from build123d import *

# Parameters (mm, degrees)
SKETCH2_W               = 7.62
SKETCH2_H               = 7.62
BOSS_EXTRUDE1_DEPTH     = 12.7
F_8_CLEARANCE_HOLE1_D   = 4.9149
CUT_EXTRUDE1_REACH      = 27.965
CUT_EXTRUDE1_END_RADIUS = 3.47345
SKETCH5_W               = 3.175
SKETCH5_H               = 3.175
CUT_EXTRUDE2_REACH      = 27.965
CUT_EXTRUDE2_END_RADIUS = 3.47345
CUT_EXTRUDE3_REACH      = 27.965
CUT_EXTRUDE3_END_RADIUS = 3.47345
SKETCH7_W               = 3.575
SKETCH7_H               = 3.575
SKETCH7_W_2             = 3.175
SKETCH7_H_2             = 3.175
CUT_EXTRUDE4_REACH      = 27.965
CUT_EXTRUDE4_END_RADIUS = 3.47345


with BuildPart() as part:
    # Sketch2 → Boss-Extrude1 (new, symmetric)
    with BuildSketch(Plane.XY):
        Rectangle(SKETCH2_W, SKETCH2_H)
    extrude(amount=BOSS_EXTRUDE1_DEPTH, both=True)

    # #8 Clearance Hole1 (through all)
    with Locations(Plane(origin=(0, 3.81, 0), x_dir=(1, 0, 0), z_dir=(0, 1, 0))):
        with Locations((0, 0)):
            Hole(F_8_CLEARANCE_HOLE1_D / 2)

    # Cut-Extrude1: up to this cylinder (the profile starts outside it)
    cut_extrude1_end = Plane(origin=(0, 0, 0), z_dir=(0, 1, 0)) * Cylinder(CUT_EXTRUDE1_END_RADIUS, 63.8769, mode=Mode.PRIVATE)
    # Sketch5 → Cut-Extrude1 (cut, up to the surface)
    with BuildSketch(Plane.XY.offset(12.7), mode=Mode.PRIVATE) as cut_extrude1_sk1:
        Rectangle(SKETCH5_W, SKETCH5_H)
    cut_extrude1_tool1 = extrude(cut_extrude1_sk1.sketch, amount=-CUT_EXTRUDE1_REACH, mode=Mode.PRIVATE) - cut_extrude1_end
    add(cut_extrude1_tool1.solids().sort_by_distance((0, 0, 12.7))[0], mode=Mode.SUBTRACT)

    # Cut-Extrude2: up to this cylinder (the profile starts outside it)
    cut_extrude2_end = Plane(origin=(0, 0, 0), z_dir=(0, 1, 0)) * Cylinder(CUT_EXTRUDE2_END_RADIUS, 63.8769, mode=Mode.PRIVATE)
    # Sketch6 → Cut-Extrude2 (cut, up to the surface)
    with BuildSketch(Plane(origin=(0, 0, -12.7), x_dir=(-1, 0, 0), z_dir=(0, 0, -1)), mode=Mode.PRIVATE) as cut_extrude2_sk1:
        with BuildLine():
            Line((1.499999936, 1.322875825), (1.499999936, -1.322875825))
            ThreePointArc((1.499999936, -1.322875825), (-2.000000064, 0), (1.499999936, 1.322875825))
        make_face()
    cut_extrude2_tool1 = extrude(cut_extrude2_sk1.sketch, amount=-CUT_EXTRUDE2_REACH, mode=Mode.PRIVATE) - cut_extrude2_end
    add(cut_extrude2_tool1.solids().sort_by_distance((0.132366, 0, -12.7))[0], mode=Mode.SUBTRACT)

    # Cut-Extrude3: up to this cylinder (the profile starts outside it)
    cut_extrude3_end = Plane(origin=(0, 0, 0), z_dir=(0, 1, 0)) * Cylinder(CUT_EXTRUDE3_END_RADIUS, 63.8769, mode=Mode.PRIVATE)
    # Sketch7 → Cut-Extrude3 (cut, up to the surface)
    with BuildSketch(Plane.XY.offset(12.7), mode=Mode.PRIVATE) as cut_extrude3_sk1:
        Rectangle(SKETCH7_W, SKETCH7_H)
        Rectangle(SKETCH7_W_2, SKETCH7_H_2, mode=Mode.SUBTRACT)
    cut_extrude3_tool1 = extrude(cut_extrude3_sk1.sketch, amount=-CUT_EXTRUDE3_REACH, mode=Mode.PRIVATE) - cut_extrude3_end
    add(cut_extrude3_tool1.solids().sort_by_distance((-1.736942, 0, 12.7))[0], mode=Mode.SUBTRACT)

    # Cut-Extrude4: up to this cylinder (the profile starts outside it)
    cut_extrude4_end = Plane(origin=(0, 0, 0), z_dir=(0, 1, 0)) * Cylinder(CUT_EXTRUDE4_END_RADIUS, 63.8769, mode=Mode.PRIVATE)
    # Sketch8 → Cut-Extrude4 (cut, up to the surface)
    with BuildSketch(Plane(origin=(0, 0, -12.7), x_dir=(-1, 0, 0), z_dir=(0, 0, -1)), mode=Mode.PRIVATE) as cut_extrude4_sk1:
        with BuildLine():
            Line((1.699999936, -1.396424183), (1.699999936, 1.396424183))
            ThreePointArc((1.699999936, 1.396424183), (-2.200000064, 0), (1.699999936, -1.396424183))
        make_face()
    cut_extrude4_tool1 = extrude(cut_extrude4_sk1.sketch, amount=-CUT_EXTRUDE4_REACH, mode=Mode.PRIVATE) - cut_extrude4_end
    add(cut_extrude4_tool1.solids().sort_by_distance((0.127385, 0, -12.7))[0], mode=Mode.SUBTRACT)


solid = part.part
Could you check a few things on this model? Use its own coordinates, in mm. A direction names the side the tool comes from. Give positions to 0.01 mm unless a question says otherwise; leave off trailing zeros. Order: outer loops, then holes, each group sorted by start corner. A loop starts at its lowest first (then second) coordinate and runs counter-clockwise, first axis right, second up. Notation, with made-up numbers: (-28, 13.25) -> (23, 13.25) arc R25 cw to (23, 45.25) -> close; hole circle Ø4 at (24, -16.5). An arc over 180 degrees is marked (long way). Answer in a Markdown table with one row per item. Add a question column.
Item 1: I'm going to push flat-ended pins straight in: P1, Ø4, axis at x = 0, z = 0, coming from the +Y side; P2, Ø3.5, axis at x = 0, y = 0, coming from the -Z side. Where does each tip first touch, or does it pass through?
Item 2: Please list where these lines run through material, in increasing order: probe 1 along X at (y, z) = (0, -6.75); probe 2 along Y at (x, z) = (0, -9); probe 3 along X at (y, z) = (-1, 6.5).
Item 3: Imagine slicing it at B-B (x = 0). List the corners of the cut face in (y, z) for me.
Item 4: We'd pull the mould along Z, two halves only. Please class faces 4 (the cylindrical face through (-1.13, -0.05, 2.18)), 5 (the flat face through (0, 3, 12.7)), 6 (the flat face through (-2, 0, -12.7)), 7 (the flat face through (3.81, 0, 0)): pulls with the +Z half, pulls with the -Z half, needs draft (parallel to the pull), parting line crosses it, or undercut.
Item 5: Imagine slicing it at C-C (z = 0). List the corners of the cut face in (x, y) for me.
Item 6: Imagine slicing it at A-A (z = 10). List the corners of the cut face in (x, y) for me, and give its area (3 significant figures).
Item 7: Imagine slicing it at D-D (y = 0). List the corners of the cut face in (x, z) for me.
Item 8: For faces 1 (the cylindrical face through (2.2, 0.08, -7.76)), 2 (the flat face through (-3, 3.81, 0)), 3 (the flat face through (1.788, 0, 8)), which set-ups out of +Z, -Z, +X, -X, +Y, -Y let a thin tool reach every point of the face, with its end or its side?
Result:
| question | item | result |
|---|---|---|
| 1 | P1 | through |
| 1 | P2 | z = -12.7 |
| 2 | probe 1 | -3.81 to -1.7, 2.2 to 3.81 |
| 2 | probe 2 | -3.81 to -2.2, 2.2 to 3.81 |
| 2 | probe 3 | -3.81 to -1.79, 1.79 to 3.81 |
| 3 | outline | (-3.81, -12.7) -> (-2.2, -12.7) -> (-2.2, -3.47) -> (2.2, -3.47) -> (2.2, -12.7) -> (3.81, -12.7) -> (3.81, -2.46) -> (-3.81, -2.46) -> close; (-3.81, 2.46) -> (3.81, 2.46) -> (3.81, 12.7) -> (1.79, 12.7) -> (1.79, 3.47) -> (-1.79, 3.47) -> (-1.79, 12.7) -> (-3.81, 12.7) -> close |
| 4 | face 4 | undercut |
| 4 | face 5 | pulls with the +Z half |
| 4 | face 6 | pulls with the -Z half |
| 4 | face 7 | needs draft |
| 5 | outline | (-3.81, -3.81) -> (-2.46, -3.81) -> (-2.46, 3.81) -> (-3.81, 3.81) -> close; (2.46, -3.81) -> (3.81, -3.81) -> (3.81, 3.81) -> (2.46, 3.81) -> close |
| 6 | outline | (-3.81, -3.81) -> (3.81, -3.81) -> (3.81, 3.81) -> (-3.81, 3.81) -> close; hole (-1.79, -1.79) -> (1.79, -1.79) -> (1.79, 1.79) -> (-1.79, 1.79) -> close |
| 6 | area | 45.3 mm2 |
| 7 | outline | (-3.81, -12.7) -> (-1.7, -12.7) -> (-1.7, -3.03) arc R3.47 ccw to (2.2, -2.69) -> (2.2, -12.7) -> (3.81, -12.7) -> (3.81, 12.7) -> (1.79, 12.7) -> (1.79, 2.98) arc R3.47 ccw to (-1.79, 2.98) -> (-1.79, 12.7) -> (-3.81, 12.7) -> close; hole circle Ø4.91 at (0, 0) |
| 8 | face 1 | -Z |
| 8 | face 2 | +Z, -Z, +X, -X, +Y |
| 8 | face 3 | +Z |
